Verification items for the finished model (mm, model axes). A direction names the side the tool comes from. Give positions to 0.01 mm unless a question says otherwise; leave off trailing zeros. Order: outer loops, then holes, each group sorted by start corner. A loop starts at its lowest first (then second) coordinate and runs counter-clockwise, first axis right, second up.
(1) Sectioned sample at C-C on x = -19.5. Record the cut outline in (y, z).
(2) Scan lines: L1, parallel to Z at x = -2.5, y = 0.45; L2, parallel to Z at x = 17, y = 0.6; L3, parallel to X at y = 1.7, z = 13.5. Record each from-to range of solid material in increasing order.
(3) Sectioned sample at B-B on z = -2.5. Record the cut outline in (x, y), plus the area to 3 significant figures.
(4) Access from +Z, -Z, +X, -X, +Y, -Y to the whole of each face (thin tool, end or side, straight path). Record for faces 1 (the face through (3, 3, -4)), 2 (the face through (15, 3, -1.5)), 3 (the face through (-21, 3, -1.5)).
(5) Mould release check, pull along Z, two halves, no side actions. Record for faces 4 (the face through (-1.5, 3, -9)), 5 (the face through (-22.5, 3, 5)), 6 (the face through (5, 3, -10)): pulls with the +Z half, pulls with the -Z half, needs draft (parallel to the pull), parting line crosses it, or undercut.
(6) Sectioned sample at A-A on z = 11.5. Record the cut outline in (x, y), plus the area to 3 significant figures.
(7) Sectioned sample at D-D on z = 4.25. Record the cut outline in (x, y).
(8) Gauge pin test, flat ends, axial feed: pin 1 (1 mm diameter, centred on y = 2.5, z = 2, fed in from +X); pin 2 (1 mm diameter, centred on x = -2, y = 2, fed in from -Z); pin 3 (2 mm diameter, centred on y = 2.5, z = -3, fed in from -X); pin 4 (12 mm diameter, centred on x = 1, z = -4, fed in from +Y). Record the tip position at first contact, or that the pin passes through.
```python
from build123d import *

# Parameters (mm, degrees)
CROQUIS1_W              = 55
CROQUIS1_H              = 30
SALIENTE_EXTRUIR1_DEPTH = 5
CORTAR_EXTRUIR1_DEPTH   = 32.721443851
CORTAR_EXTRUIR2_DEPTH   = 32.721443851
CORTAR_EXTRUIR3_DEPTH   = 32.721443851


with BuildPart() as part:
    # Croquis1 → Saliente-Extruir1 (new body)
    with BuildSketch(Plane(origin=(0, 0, 0), x_dir=(1, 0, 0), z_dir=(0, 1, 0))):
        Rectangle(CROQUIS1_W, CROQUIS1_H)
    extrude(amount=SALIENTE_EXTRUIR1_DEPTH)

    # Croquis2 → Cortar-Extruir1 (cut, through all)
    with BuildSketch(Plane(origin=(0, 5, 0), x_dir=(1, 0, 0), z_dir=(0, 1, 0))):
        Polygon((-22.5, 8), (-27.5, 8), (-27.5, -8), (-22.5, -8), (-22.5, -1.5), (-20.5, -1.5), (-20.5, -3.5), (-16.5, -3.5), (-16.5, -1.5), (-13.5, -1.5), (-13.5, 1.5), (-16.5, 1.5), (-16.5, 3.5), (-20.5, 3.5), (-20.5, 1.5), (-22.5, 1.5), align=None)
    cortar_extruir1 = extrude(amount=-CORTAR_EXTRUIR1_DEPTH, mode=Mode.SUBTRACT)

    # Simetría1: Cortar-Extruir1 across plane
    add(cortar_extruir1.mirror(Plane(origin=(0, 0, 0), x_dir=(0, 0, 1), z_dir=(1, 0, 0))), mode=Mode.SUBTRACT)

    # Croquis3 → Cortar-Extruir2 (cut, through all)
    with BuildSketch(Plane(origin=(0, 5, 0), x_dir=(1, 0, 0), z_dir=(0, 1, 0))):
        Polygon((-8, 15), (8, 15), (8, 10), (1.5, 10), (1.5, 8), (3.5, 8), (3.5, 4), (1.5, 4), (1.5, 1), (-1.5, 1), (-1.5, 4), (-3.5, 4), (-3.5, 8), (-1.5, 8), (-1.5, 10), (-8, 10), align=None)
    extrude(amount=-CORTAR_EXTRUIR2_DEPTH, mode=Mode.SUBTRACT)

    # Croquis4 → Cortar-Extruir3 (cut, through all)
    with BuildSketch(Plane(origin=(0, 5, 0), x_dir=(1, 0, 0), z_dir=(0, 1, 0))):
        Polygon((1.5, -15), (1.5, -13), (3.5, -13), (3.5, -9), (1.5, -9), (1.5, -6), (-1.5, -6), (-1.5, -9), (-3.5, -9), (-3.5, -13), (-1.5, -13), (-1.5, -15), align=None)
    extrude(amount=-CORTAR_EXTRUIR3_DEPTH, mode=Mode.SUBTRACT)


solid = part.part
```
Ans:
1. outline: (0, -15) - (5, -15) - (5, -3.5) - (0, -3.5) - close; (0, 3.5) - (5, 3.5) - (5, 15) - (0, 15) - close
2. L1: z = -10 to -8, -4 to 9, 13 to 15
2. L2: z = -15 to -3.5, 3.5 to 15
2. L3: x = -27.5 to -1.5, 1.5 to 27.5
3. outline: (-22.5, 0) - (-20.5, 0) - (-20.5, 5) - (-22.5, 5) - close; (-16.5, 0) - (-1.5, 0) - (-1.5, 5) - (-16.5, 5) - close; (1.5, 0) - (16.5, 0) - (16.5, 5) - (1.5, 5) - close; (20.5, 0) - (22.5, 0) - (22.5, 5) - (20.5, 5) - close
3. area: 170 mm2
4. face 1: +Y, -Y
4. face 2: +X, +Y, -Y
4. face 3: -X, +Y, -Y
5. face 4: needs draft
5. face 5: undercut
5. face 6: pulls with the -Z half
6. outline: (-27.5, 0) - (-3.5, 0) - (-3.5, 5) - (-27.5, 5) - close; (3.5, 0) - (27.5, 0) - (27.5, 5) - (3.5, 5) - close
6. area: 240 mm2
7. outline: (-22.5, 0) - (22.5, 0) - (22.5, 5) - (-22.5, 5) - close
8. pin 1: stops at x = 22.5
8. pin 2: stops at z = -10
8. pin 3: stops at x = -22.5
8. pin 4: stops at y = 5
